from build123d import *

# Parameters (mm, degrees)
BOSS_EXTRUDE1_DEPTH    = 6.35
F_10_CLEARANCE_HOLE1_D = 5.6134


with BuildPart() as part:
    # Sketch1 → Boss-Extrude1 (new body)
    with BuildSketch(Plane.XY):
        Polygon((-533.470529443, 0), (533.470529443, 0), (438.15, 165.1), (-438.15, 165.1), align=None)
    extrude(amount=BOSS_EXTRUDE1_DEPTH)

    # #10 Clearance Hole1 (through all)
    with Locations(Plane.XY.offset(6.35)):
        with Locations((-50.8, 19.05), (50.8, 19.05)):
            Hole(F_10_CLEARANCE_HOLE1_D / 2)


solid = part.part
Model file for the job. Use its own axes, mm. Round coordinates to 2 decimals unless told otherwise and drop trailing zeros. Order: outer loops, then holes, each group sorted by start corner. A loop starts at its lowest first (then second) coordinate and runs counter-clockwise, first axis right, second up.
(1) Drill centre lines: line 1 (Y direction, x = 50.8, z = 3.5); line 2 (X direction, y = 112.5, z = 4.75); line 3 (Y direction, x = 461, z = 3.75). Where is each one in solid material? Low to high.
(2) Band-saw the part on C-C (y = 36). List the corners of the cut face in (x, z), then the cut area to 3 significant figures.
(3) Band-saw the part on A-A (z = 2.75). List the corners of the cut face in (x, y).
(4) Pin check, flat tips, straight feed: pin 1 (3 mm diameter, centred on y = 130.5, z = 1, fed in from +X); pin 2 (1 mm diameter, centred on y = 102.5, z = 4.5, fed in from -X). Stop position of each tip, or through.
(5) Band-saw the part on B-B (y = 76). List the corners of the cut face in (x, z), then the cut area to 3 significant figures.
Verdict:
1. line 1: y = 0 to 16.24, 21.86 to 165.1
1. line 2: x = -468.52 to 468.52
1. line 3: y = 0 to 125.52
2. outline: (-512.69, 0) - (512.69, 0) - (512.69, 6.35) - (-512.69, 6.35) - close
2. area: 6,510 mm2
3. outline: (-533.47, 0) - (533.47, 0) - (438.15, 165.1) - (-438.15, 165.1) - close; hole circle Ø5.61 at (-50.8, 19.05); hole circle Ø5.61 at (50.8, 19.05)
4. pin 1: stops at x = 458.99
4. pin 2: stops at x = -474.58
5. outline: (-489.59, 0) - (489.59, 0) - (489.59, 6.35) - (-489.59, 6.35) - close
5. area: 6,220 mm2
